Verification items for the finished model (mm, model axes). Face numbers are marked on the shaded views. A direction names the side the tool comes from. Give positions to 0.01 mm unless a question says otherwise; leave off trailing zeros. Order: outer loops, then holes, each group sorted by start corner. A loop starts at its lowest first (then second) coordinate and runs counter-clockwise, first axis right, second up.
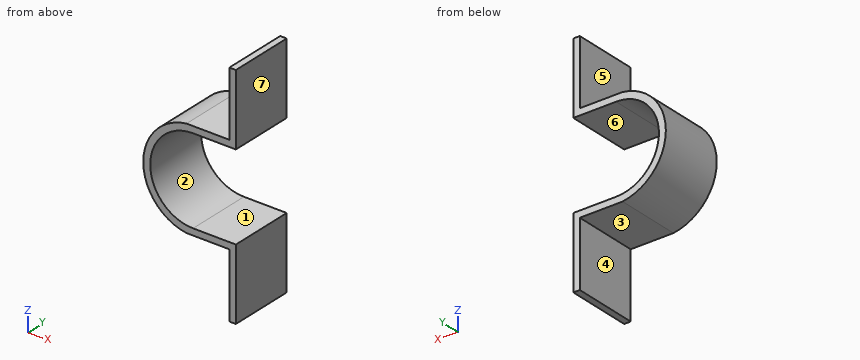
Autodesk Inventor part; units mm, degrees
ref_plane "YZ Plane" through (0, 0, 0) normal (1, 0, 0) x (0, 1, 0)
ref_plane "XZ Plane" through (0, 0, 0) normal (0, 1, 0) x (-1, 0, 0)
ref_plane "XY Plane" through (0, 0, 0) normal (0, 0, 1) x (1, 0, 0)
sketch "Sketch1" plane through (0, 0, 0) normal (0, 1, 0) x (-1, 0, 0)
  arc A0 (0, -21.6252) -> (0, 11.7758) centre (0, -4.9247) ccw
  line L0 (0, 37.1885) -> (0, 11.7885)
  line L1 (0, -21.6379) -> (0, -47.0379)
  arc A1 (0, -21.6379) -> (0, 11.7885) centre (0, -4.9247) ccw
  line L2 (0, 37.1885) -> (2.54, 37.1885)
  line L3 (0, -47.0379) -> (2.54, -47.0379)
  line L4 (2.54, 37.1885) -> (2.54, 14.3285)
  line L5 (2.54, -47.0379) -> (2.54, -24.1779)
  arc A2 (2.54, -24.1779) -> (2.54, 14.3285) centre (0, -4.9247) ccw
  dimension "d0" = 33.401
  dimension "d1" = 25.4
  dimension "d2" = 25.4
  dimension "d3" = 33.4264
  dimension "d6" = 16.7132
  dimension "d7" = 16.7132
  dimension "d8" = 2.54
  dimension "d9" = 2.54
  dimension "d10" = 19.2532
  dimension "d11" = 19.2532
extrude "Extrusion1" add sketch "Sketch1" along normal blind 25.4
sketch "Sketch2" plane through (0, 0, 37.1885) normal (1, 0, 0) x (0, 0, -1)
  line L0 (25.4, 0) -> (25.4, 25.4)
  line L1 (22.86, 0) -> (22.86, 25.4)
  line L2 (25.4, 25.4) -> (22.86, 25.4)
  line L3 (22.86, 25.4) -> (22.86, 0)
  line L4 (22.86, 0) -> (25.4, 0)
  line L5 (25.4, 0) -> (25.4, 25.4)
  line L6 (25.4, 25.4) -> (58.8264, 25.4)
  line L7 (61.3664, 0) -> (22.86, 0)
  line L8 (58.8264, 25.4) -> (61.3664, 25.4)
  line L9 (61.3664, 25.4) -> (61.3664, 0)
  line L10 (61.3664, 0) -> (58.8264, 0)
  line L11 (58.8264, 0) -> (58.8264, 25.4)
  point P0 (37.1885, 0)
extrude "Extrusion2" add sketch "Sketch2" along normal blind 16.7005 contours L4 L1 L2 L0 | L11 L8 L9 L7
sketch "Sketch3" plane through (0, 0, -47.0379) normal (1, 0, 0) x (0, 0, -1)
  line L0 (0, 25.4) -> (-22.86, 25.4)
  line L1 (-22.86, 0) -> (0, 0)
  line L2 (0, 25.4) -> (-22.86, 25.4)
  line L3 (-22.86, 25.4) -> (-22.86, 0)
  line L4 (-22.86, 0) -> (0, 0)
  line L5 (0, 0) -> (0, 25.4)
  line L6 (-61.3664, 25.4) -> (-84.2264, 25.4)
  line L7 (-22.86, 0) -> (-61.3664, 0)
  line L8 (-84.2264, 25.4) -> (-61.3664, 25.4)
  line L9 (-61.3664, 25.4) -> (-61.3664, 0)
  line L10 (-61.3664, 0) -> (-84.2264, 0)
  line L11 (-84.2264, 0) -> (-84.2264, 25.4)
  point P0 (-47.0379, 0)
extrude "Extrusion3" cut sketch "Sketch3" against normal blind 16.7005
sketch "Sketch4" plane through (16.7005, 25.4, -24.1779) normal (0, 0, -1) x (-1, 0, 0)
  line L0 (0, -25.4) -> (0, 0)
  line L1 (16.7005, 0) -> (0, 0)
  line L2 (0, -25.4) -> (2.54, -25.4)
  line L3 (2.54, -25.4) -> (2.54, 0)
  line L4 (2.54, 0) -> (0, 0)
  line L5 (0, 0) -> (0, -25.4)
  point P0 (16.7005, -25.4)
  dimension "d18" = 2.54
extrude "Extrusion4" add sketch "Sketch4" along normal blind 25.4
sketch "Sketch5" plane through (-2.54, 0, 14.3285) normal (0, 0, 1) x (1, 0, 0)
  line L0 (19.2405, 25.4) -> (19.2405, 0)
  line L1 (16.7005, 0) -> (16.7005, 25.4)
  line L2 (19.2405, 0) -> (16.7005, 0)
  line L3 (16.7005, 0) -> (16.7005, 25.4)
  line L4 (16.7005, 25.4) -> (19.2405, 25.4)
  line L5 (19.2405, 25.4) -> (19.2405, 0)
  point P0 (2.54, 0)
extrude "Extrusion5" add sketch "Sketch5" along normal blind 25.4
equation "\"d2\" = d1"
equation "\"d7\" = d6"
equation "\"d9\" = d8"
properties part number "Attachy-thing Derek"
(1) Section check C-C, the plane x = -3.5. Enter the section's corners in (y, z), then the cut area to 3 significant figures.
Solved:
outline: (0, -24.03) - (25.4, -24.03) - (25.4, -21.27) - (0, -21.27) - close; (0, 11.42) - (25.4, 11.42) - (25.4, 14.18) - (0, 14.18) - close
area: 140 mm2
(2) Release check for a two-part mould opening along Z. For the marked faces 1, 2, 3 and 4 record: pulls with the +Z half, pulls with the -Z half, needs draft (parallel to the pull), parting line crosses it, or undercut.
Solved:
face 1: undercut
face 2: undercut
face 3: pulls with the -Z half
face 4: needs draft
(3) Go/stop test with flat-tipped pins: pin 1 (5 mm diameter, centred on x = 11, y = 6.5, fed in from +Z); pin 2 (2 mm diameter, centred on x = 3.5, y = 22, fed in from -Z); pin 3 (8 mm diameter, centred on y = 13.5, z = -31.5, fed in from -X); pin 4 (12 mm diameter, centred on y = 20.5, z = -19, fed in from +X). Record where each tip stops, or that it passes through.
Solved:
pin 1: stops at z = 14.33
pin 2: stops at z = -24.18
pin 3: stops at x = 14.16
pin 4: stops at x = 16.7
(4) Section check A-A, the plane x = 7.5. Enter the section's corners in (y, z).
Solved:
outline: (0, -24.18) - (25.4, -24.18) - (25.4, -21.64) - (0, -21.64) - close; (0, 11.79) - (25.4, 11.79) - (25.4, 14.33) - (0, 14.33) - close
(5) Scan lines: line 1 (Z direction, x = 4.5, y = 18.75); line 2 (X direction, y = 18.5, z = -37); line 3 (Z direction, x = -13.5, y = 13.25). Record each from-to range of solid material in increasing order.
Solved:
line 1: z = -24.18 to -21.64, 11.79 to 14.33
line 2: x = 14.16 to 16.7
line 3: z = -18.88 to -14.78, 4.93 to 9.04
(6) Set-up check for the marked faces 5, 6 and 7: record each of +Z, -Z, +X, -X, +Y, -Y from which the full face is reachable in a straight line by a thin tool's end or side.
Solved:
face 5: +Z, -X, +Y, -Y
face 6: +X, +Y, -Y
face 7: +Z, -Z, +X, +Y, -Y
(7) Section check D-D, the plane z = 18. Enter the section's corners in (x, y).
Solved:
outline: (14.16, 0) - (16.7, 0) - (16.7, 25.4) - (14.16, 25.4) - close
(8) Section check B-B, the plane y = 14.75. Enter the section's corners in (x, z).
Solved:
outline: (-2.54, -24.18) - (14.16, -24.18) - (14.16, -49.58) - (16.7, -49.58) - (16.7, -21.64) - (0, -21.64) arc R16.71 cw to (0, 11.79) - (16.7, 11.79) - (16.7, 39.73) - (14.16, 39.73) - (14.16, 14.33) - (-2.54, 14.33) arc R19.42 ccw to start
